The listing builds one solid part. Answer for the finished solid, in the listing's coordinates (mm). Face numbers are marked on the shaded views. A direction names the side the tool comes from. Give positions to 0.01 mm unless a question says otherwise; leave off trailing zeros. Loops run counter-clockwise (first coordinate to the right, second up) from the corner with the lowest first, then second, coordinate; pieces in that order, holes last. Notation, with made-up numbers: (-36.5, 5) - (18.5, 5) arc R24 cw to (18.5, 39) - close; hole circle Ø5 at (66, -28.5). An arc over 180 degrees is marked (long way). Answer in a Markdown table with one row per item. Add a question column.
```python
from build123d import *

# Parameters (mm, degrees)
SKETCH_1_W               = 53
SKETCH_1_H               = 30.25
EXTRUDE_1_DEPTH          = 32
SKETCH_2_W               = 49
SKETCH_2_H               = 26.25
CUT_EXTRUDE_1_DEPTH      = 24
SKETCH_3_W               = 52
SKETCH_3_H               = 29.25
SKETCH_3_W_2             = 50.4
SKETCH_3_H_2             = 27.65
CUT_EXTRUDE_2_DEPTH      = 1
EXTRUDE_2_DEPTH          = 15
SKETCH_7_R               = 1
CUT_EXTRUDE_4_DEPTH      = 10
MIRROR_2_COPY_1_DEPTH    = 15
MIRROR_2_COPY_2_SKETCH_R = 1
MIRROR_2_COPY_2_DEPTH    = 10
SKETCH_8_W               = 53
SKETCH_8_H               = 30.25
CUT_EXTRUDE_5_DEPTH      = 2
SKETCH_11_R              = 5
CUT_EXTRUDE_6_DEPTH      = 43.790368367
SKETCH_12_R              = 11.5
SKETCH_12_R_2            = 9.5
EXTRUDE_4_DEPTH          = 5
CUT_EXTRUDE_START        = -4.5
SKETCH_13_R              = 9.5
CUT_EXTRUDE_7_DEPTH      = 4.5
SKETCH_14_W              = 53
SKETCH_14_H              = 30.25
SKETCH_14_R              = 11.5
CUT_EXTRUDE_8_DEPTH      = 4.5
SKETCH_15_R              = 2
SKETCH_15_R_2            = 1
EXTRUDE_5_DEPTH          = 3
SKETCH_16_R              = 2
SKETCH_16_R_2            = 1
EXTRUDE_6_DEPTH          = 3
EXTRUDE_START            = 2
SKETCH_18_R              = 11.5
SKETCH_18_R_2            = 7
EXTRUDE_8_DEPTH          = 2
SKETCH_19_R              = 11.5
SKETCH_19_R_2            = 5
EXTRUDE_9_DEPTH          = 2


with BuildPart() as part:
    # 草图1 → 凸台-拉伸1 (new body)
    with BuildSketch(Plane.XY):
        Rectangle(SKETCH_1_W, SKETCH_1_H)
    extrude(amount=EXTRUDE_1_DEPTH)

    # 草图2 → 切除-拉伸1 (cut)
    with BuildSketch(Plane.XY.offset(32)):
        Rectangle(SKETCH_2_W, SKETCH_2_H)
    extrude(amount=-CUT_EXTRUDE_1_DEPTH, mode=Mode.SUBTRACT)

    # 草图3 → 切除-拉伸2 (cut)
    with BuildSketch(Plane.XY.offset(32)):
        Rectangle(SKETCH_3_W, SKETCH_3_H)
        Rectangle(SKETCH_3_W_2, SKETCH_3_H_2, mode=Mode.SUBTRACT)
    extrude(amount=-CUT_EXTRUDE_2_DEPTH, mode=Mode.SUBTRACT)

    # 草图6 → 凸台-拉伸2 (add)
    with BuildSketch(Plane.XY.offset(8)):
        with BuildLine():
            Line((-22.656269654, 13.125), (-24.5, 13.125))
            Line((-24.5, 13.125), (-24.5, 11.268730346))
            ThreePointArc((-24.5, 11.268730346), (-21.33741914, 9.97128577), (-22.656269654, 13.125))
        make_face()
    extrude_2 = extrude(amount=EXTRUDE_2_DEPTH)

    # 草图7 → 切除-拉伸4 (cut)
    with BuildSketch(Plane.XY.offset(23)):
        with Locations((-22.65, 11.275)):
            Circle(SKETCH_7_R)
    cut_extrude_4 = extrude(amount=-CUT_EXTRUDE_4_DEPTH, mode=Mode.SUBTRACT)

    # 镜向1: 凸台-拉伸2, 切除-拉伸4 across plane
    add(extrude_2.mirror(Plane.ZX))
    add(cut_extrude_4.mirror(Plane.ZX), mode=Mode.SUBTRACT)

    # 镜向2: 凸台-拉伸2, 切除-拉伸4 across plane
    add(extrude_2.mirror(Plane(origin=(0, 0, 0), x_dir=(0, 0, 1), z_dir=(1, 0, 0))))
    add(cut_extrude_4.mirror(Plane(origin=(0, 0, 0), x_dir=(0, 0, 1), z_dir=(1, 0, 0))), mode=Mode.SUBTRACT)

    # 镜向2 copy 1 sketch → 镜向2 copy 1 (add)
    with BuildSketch(Plane(origin=(0, 0, 8), x_dir=(-1, 0, 0), z_dir=(0, 0, 1))):
        with BuildLine():
            Line((-22.656269654, 13.125), (-24.5, 13.125))
            Line((-24.5, 13.125), (-24.5, 11.268730346))
            ThreePointArc((-24.5, 11.268730346), (-21.33741914, 9.97128577), (-22.656269654, 13.125))
        make_face()
    extrude(amount=MIRROR_2_COPY_1_DEPTH)

    # 镜向2 copy 2 sketch → 镜向2 copy 2 (cut)
    with BuildSketch(Plane(origin=(0, 0, 23), x_dir=(-1, 0, 0), z_dir=(0, 0, 1))):
        with Locations((-22.65, 11.275)):
            Circle(MIRROR_2_COPY_2_SKETCH_R)
    extrude(amount=-MIRROR_2_COPY_2_DEPTH, mode=Mode.SUBTRACT)

    # 草图8 → 切除-拉伸5 (cut)
    with BuildSketch(Plane(origin=(0, 0, 0), x_dir=(-1, 0, 0), z_dir=(0, 0, -1))):
        Rectangle(SKETCH_8_W, SKETCH_8_H)
    extrude(amount=-CUT_EXTRUDE_5_DEPTH, mode=Mode.SUBTRACT)

    # 草图11 → 切除-拉伸6 (cut, through all)
    with BuildSketch(Plane(origin=(0, 0, 2), x_dir=(-1, 0, 0), z_dir=(0, 0, -1))):
        with Locations((-12.7, 0)):
            Circle(SKETCH_11_R)
    extrude(amount=-CUT_EXTRUDE_6_DEPTH, mode=Mode.SUBTRACT)

    # 草图12 → 凸台-拉伸4 (add)
    with BuildSketch(Plane.XY.offset(8)):
        with Locations((12.7, 0)):
            Circle(SKETCH_12_R)
        with Locations((12.7, 0)):
            Circle(SKETCH_12_R_2, mode=Mode.SUBTRACT)
    extrude(amount=EXTRUDE_4_DEPTH)

    # 草图13 → 切除-拉伸7 (cut)
    with BuildSketch(Plane.XY.offset(8).offset(CUT_EXTRUDE_START)):
        with Locations((12.7, 0)):
            Circle(SKETCH_13_R)
    extrude(amount=CUT_EXTRUDE_7_DEPTH, mode=Mode.SUBTRACT)

    # 草图14 → 切除-拉伸8 (cut)
    with BuildSketch(Plane(origin=(0, 0, 2), x_dir=(-1, 0, 0), z_dir=(0, 0, -1))):
        Rectangle(SKETCH_14_W, SKETCH_14_H)
        with Locations(Location((-12.7, 0, 0), (0, 0, 180))):
            Circle(SKETCH_14_R, mode=Mode.SUBTRACT)
    extrude(amount=-CUT_EXTRUDE_8_DEPTH, mode=Mode.SUBTRACT)

    # 草图15 → 凸台-拉伸5 (add)
    with BuildSketch(Plane.XY.offset(8)):
        with Locations((-12.5, 0.005)):
            Circle(SKETCH_15_R)
        with Locations((-12.5, 0.005)):
            Circle(SKETCH_15_R_2, mode=Mode.SUBTRACT)
    extrude(amount=EXTRUDE_5_DEPTH)

    # 草图16 → 凸台-拉伸6 (add)
    with BuildSketch(Plane.XY.offset(8)):
        Circle(SKETCH_16_R)
        Circle(SKETCH_16_R_2, mode=Mode.SUBTRACT)
    extrude(amount=EXTRUDE_6_DEPTH)

    # 草图18 → 凸台-拉伸8 (add)
    with BuildSketch(Plane(origin=(0, 0, 2), x_dir=(-1, 0, 0), z_dir=(0, 0, -1)).offset(EXTRUDE_START)):
        with Locations(Location((-12.7, 0, 0), (0, 0, 7.591184195))):
            Circle(SKETCH_18_R)
        with Locations((-12.7, 0)):
            Circle(SKETCH_18_R_2, mode=Mode.SUBTRACT)
    extrude(amount=-EXTRUDE_8_DEPTH)

    # 草图19 → 凸台-拉伸9 (add)
    with BuildSketch(Plane(origin=(0, 0, 0), x_dir=(-1, 0, 0), z_dir=(0, 0, -1)).offset(EXTRUDE_START)):
        with Locations(Location((-12.7, 0, 0), (0, 0, 7.591184195))):
            Circle(SKETCH_19_R)
        with Locations((-12.7, 0)):
            Circle(SKETCH_19_R_2, mode=Mode.SUBTRACT)
    extrude(amount=-EXTRUDE_9_DEPTH)


solid = part.part
```
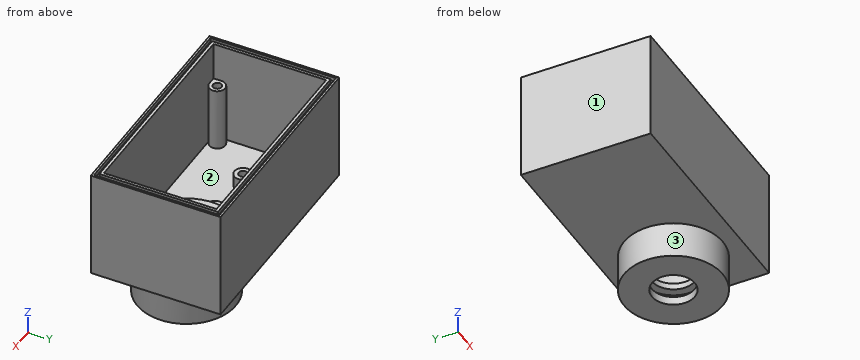
(1) Given pin 1 Ø13 at (x, y) = (-3, 1.5) entering from +Z; pin 2 Ø2 at (x, z) = (-17.5, 4.5) entering from +Y; pin 3 Ø9 at (x, y) = (-11.5, 3.5) entering from +Z; pin 4 Ø8 at (y, z) = (-8, 1.5) entering from -X, each flat-ended and moving along its own axis, determine where each tip first touches the part or whether it passes through.
(2) A cutting plane is placed at C-C on z = 19. Determine the outline of the cut face in (x, y) (3 decimals).
(3) A cutting plane is placed at B-B on x = -12.5. Determine the outline of the cut face in (y, z) (3 decimals), plus the area to 3 significant figures.
(4) A cutting plane is placed at D-D on x = 4. Determine the outline of the cut face in (y, z) (3 decimals).
(5) Find the intervals of material crossed by line 1 along Y through (x, z) = (0, 9) (3 decimals); line 2 along X through (y, z) = (-5, 21); line 3 along Y through (x, z) = (-23.5, 22) (3 decimals), in increasing order. Write a range as [from, to].
(6) A tool of negligible diameter and unlimited length cuts with its end or side. For the marked faces 1, 2 and 3, from which of +Z, -Z, +X, -X, +Y, -Y can it reach the whole face along a straight path? Write none if from no direction.
(7) A cutting plane is placed at A-A on z = 25. Determine the outline of the cut face in (x, y) (3 decimals), plus the area to 3 significant figures.
Evaluation:
| question | item | result |
|---|---|---|
| 1 | pin 1 | stops at z = 13 |
| 1 | pin 2 | passes through |
| 1 | pin 3 | stops at z = 11 |
| 1 | pin 4 | stops at x = 1.92 |
| 2 | outline | (-26.5, -15.125) - (26.5, -15.125) - (26.5, 15.125) - (-26.5, 15.125) - close; hole (-24.5, -11.269) arc R1.85 cw (long way) to (-22.644, -13.125) - (22.644, -13.125) arc R1.85 cw (long way) to (24.5, -11.269) - (24.5, 11.269) arc R1.85 cw (long way) to (22.644, 13.125) - (-22.644, 13.125) arc R1.85 cw (long way) to (-24.5, 11.269) - close; hole circle Ø2 at (-22.65, -11.275); hole circle Ø2 at (-22.65, 11.275); hole circle Ø2 at (22.65, -11.275); hole circle Ø2 at (22.65, 11.275) |
| 3 | outline | (-15.125, 6.5) - (15.125, 6.5) - (15.125, 32) - (14.625, 32) - (14.625, 31) - (13.825, 31) - (13.825, 32) - (13.125, 32) - (13.125, 8) - (2.005, 8) - (2.005, 11) - (1.005, 11) - (1.005, 8) - (-0.995, 8) - (-0.995, 11) - (-1.995, 11) - (-1.995, 8) - (-13.125, 8) - (-13.125, 32) - (-13.825, 32) - (-13.825, 31) - (-14.625, 31) - (-14.625, 32) - (-15.125, 32) - close |
| 3 | area | 146 mm² |
| 4 | outline | (-15.125, 6.5) - (-7.521, 6.5) - (-7.521, -2) - (7.521, -2) - (7.521, 6.5) - (15.125, 6.5) - (15.125, 32) - (14.625, 32) - (14.625, 31) - (13.825, 31) - (13.825, 32) - (13.125, 32) - (13.125, 8) - (7.521, 8) - (7.521, 13) - (3.816, 13) - (3.816, 3.5) - (-3.816, 3.5) - (-3.816, 13) - (-7.521, 13) - (-7.521, 8) - (-13.125, 8) - (-13.125, 32) - (-13.825, 32) - (-13.825, 31) - (-14.625, 31) - (-14.625, 32) - (-15.125, 32) - close |
| 5 | line 1 | y = [-15.125, -13.125], [-2, -1], [1, 2], [13.125, 15.125] |
| 5 | line 2 | x = [-26.5, -24.5], [24.5, 26.5] |
| 5 | line 3 | y = [-15.125, -11.802], [-10.748, -9.632], [9.632, 10.748], [11.802, 15.125] |
| 6 | face 1 | +Z, -Z, -X, +Y, -Y |
| 6 | face 2 | +Z |
| 6 | face 3 | -Z |
| 7 | outline | (-26.5, -15.125) - (26.5, -15.125) - (26.5, 15.125) - (-26.5, 15.125) - close; hole (-24.5, -13.125) - (24.5, -13.125) - (24.5, 13.125) - (-24.5, 13.125) - close |
| 7 | area | 317 mm² |
